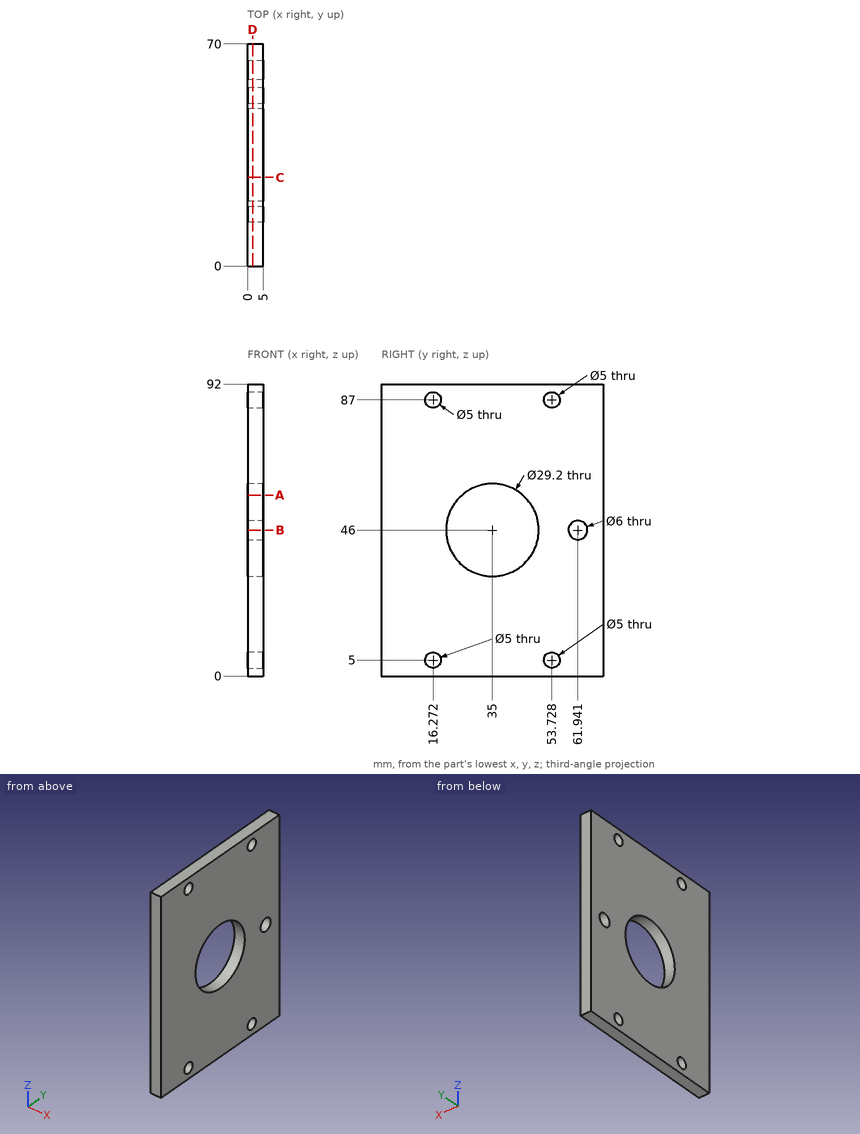
Answer from the drawing. Dimensions are ordinates in mm from the lowest x, y and z of the part. Give positions to 0.01 mm unless a question says otherwise; leave off trailing zeros. Loops run counter-clockwise (first coordinate to the right, second up) from the corner with the lowest first, then second, coordinate; pieces in that order, holes last. Notation, with made-up numbers: (29, 58.5) - (33, 58.5) arc R27 ccw to (33, 92.5) - close; hole circle Ø8 at (32, 3). An arc over 180 degrees is marked (long way). Answer as CSV lines item,"result". Start each with the question number.
Item 1: A cutting plane is placed at B-B on z = 46. Determine the outline of the cut face in (x, y).
Item 2: A cutting plane is placed at A-A on z = 57. Determine the outline of the cut face in (x, y).
Item 3: This flat-tipped pin is pushed along its axis until it touches: pin 1 (6 mm diameter, centred on y = 16.27, z = 5, fed in from -X). Where does it stop, or does it pass through?
Item 4: A cutting plane is placed at D-D on x = 1.6. Determine the outline of the cut face in (y, z), then the cut area to 3 significant figures.
Item 5: Find the intervals of material crossed by line 1 (Y direction, x = 2.3, z = 46); line 2 (Y direction, x = 3.25, z = 5); line 3 (Z direction, x = 2.75, y = 55), in increasing order. Write a range as from..to.
Item 6: A cutting plane is placed at C-C on y = 28. Determine the outline of the cut face in (x, z), then the cut area to 3 significant figures.
Found:
1,outline,"(0, 0) - (5, 0) - (5, 20.4) - (0, 20.4) - close; (0, 49.6) - (5, 49.6) - (5, 58.94) - (0, 58.94) - close; (0, 64.94) - (5, 64.94) - (5, 70) - (0, 70) - close"
2,outline,"(0, 0) - (5, 0) - (5, 25.4) - (0, 25.4) - close; (0, 44.6) - (5, 44.6) - (5, 70) - (0, 70) - close"
3,pin 1,"stops at x = 0"
4,outline,"(0, 0) - (70, 0) - (70, 92) - (0, 92) - close; hole circle Ø5 at (16.27, 5); hole circle Ø5 at (16.27, 87); hole circle Ø29.2 at (35, 46); hole circle Ø5 at (53.73, 5); hole circle Ø5 at (53.73, 87); hole circle Ø6 at (61.94, 46)"
4,area,"5,660 mm^2"
5,line 1,"y = 0..20.4, 49.6..58.94, 64.94..70"
5,line 2,"y = 0..13.77, 18.77..51.23, 56.23..70"
5,line 3,"z = 0..2.85, 7.15..84.85, 89.15..92"
6,outline,"(0, 0) - (5, 0) - (5, 33.19) - (0, 33.19) - close; (0, 58.81) - (5, 58.81) - (5, 92) - (0, 92) - close"
6,area,"332 mm^2"
